Geometry check sheet. Reference: the model listing, model coordinates, mm. A direction names the side the tool comes from. Round coordinates to 2 decimals unless told otherwise and drop trailing zeros. Write each loop counter-clockwise with the first axis right and the second up, starting at its lowest first coordinate (ties: lowest second). Pieces come first, ordered by that corner, then holes.
Item 1: Draft check along Z on faces 3 (the face through (3.5, 0, 6)), 4 (the face through (0.08, -3.51, 5.75)), 5 (the face through (-2.4, 0.1, 0)). Enter one of: pulls with the +Z half, pulls with the -Z half, needs draft (parallel to the pull), parting line crosses it, or undercut.
Item 2: Access from +Z, -Z, +X, -X, +Y, -Y to the whole of each face (thin tool, end or side, straight path). Record for faces 1 (the face through (0, 4, 6)), 2 (the face through (0, -3, 4)).
Item 3: Cross-section at B-B (x = 0). Enter the section's corners in (y, z).
Item 4: Cross-section at D-D (y = 2). Enter the section's corners in (x, z).
Item 5: Cross-section at A-A (y = 0). Enter the section's corners in (x, z), then the cut area to 3 significant figures.
Item 6: Cross-section at C-C (z = 12). Enter the section's corners in (x, y).
Item 7: Depth check by flat-ended pin: P1, Ø2, axis at x = 0, z = 4, coming from the -Y side. Enter the tip coordinate at first touch or a pass-through.
Item 8: Scan lines: probe 1 along X at (y, z) = (-3.65, 4); probe 2 along X at (y, z) = (-0.75, 11.5); probe 3 along Y at (x, z) = (0, 5.25). Record each from-to range of solid material in increasing order.
from build123d import *

# Parameters (mm, degrees)
ESQUISSE1_W             = 7
ESQUISSE1_H             = 8
ESQUISSE1_R             = 2.25
BOSS_EXTRU_1_DEPTH      = 13
ESQUISSE2_R             = 1.75
ENL_V_MAT_EXTRU_1_DEPTH = 1


with BuildPart() as part:
    # Esquisse1 → Boss.-Extru.1 (new body)
    with BuildSketch(Plane.XY):
        Rectangle(ESQUISSE1_W, ESQUISSE1_H)
        with Locations(Location((0, 0, 0), (0, 0, 180))):
            Circle(ESQUISSE1_R, mode=Mode.SUBTRACT)
    extrude(amount=BOSS_EXTRU_1_DEPTH)

    # Esquisse2 → Enlèv. mat.-Extru.1 (cut)
    with BuildSketch(Plane.XZ.offset(4)):
        with Locations(Location((0, 4, 0), (0, 0, 270))):
            Circle(ESQUISSE2_R)
    extrude(amount=-ENL_V_MAT_EXTRU_1_DEPTH, mode=Mode.SUBTRACT)


solid = part.part
Resolved:
1. face 3: needs draft
1. face 4: undercut
1. face 5: pulls with the -Z half
2. face 1: +Z, -Z, +X, -X, +Y
2. face 2: -Y
3. outline: (-4, 0) - (-2.25, 0) - (-2.25, 13) - (-4, 13) - (-4, 5.75) - (-3, 5.75) - (-3, 2.25) - (-4, 2.25) - close; (2.25, 0) - (4, 0) - (4, 13) - (2.25, 13) - close
4. outline: (-3.5, 0) - (-1.03, 0) - (-1.03, 13) - (-3.5, 13) - close; (1.03, 0) - (3.5, 0) - (3.5, 13) - (1.03, 13) - close
5. outline: (-3.5, 0) - (-2.25, 0) - (-2.25, 13) - (-3.5, 13) - close; (2.25, 0) - (3.5, 0) - (3.5, 13) - (2.25, 13) - close
5. area: 32.5 mm2
6. outline: (-3.5, -4) - (3.5, -4) - (3.5, 4) - (-3.5, 4) - close; hole circle Ø4.5 at (0, 0)
7. P1: stops at y = -3
8. probe 1: x = -3.5 to -1.75, 1.75 to 3.5
8. probe 2: x = -3.5 to -2.12, 2.12 to 3.5
8. probe 3: y = -3 to -2.25, 2.25 to 4
